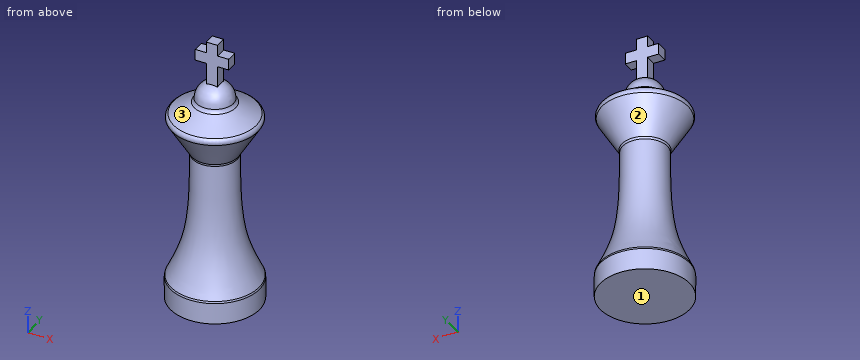
from build123d import *

# Parameters (mm, degrees)
F0_W     = 5
F0_H     = 20
F1_DEPTH = 2.5
F2_W     = 15
F2_H     = 5
F3_DEPTH = 2.5
F6_DEPTH = 2.5
F7_DEPTH = 5
F8_R     = 2


with BuildPart() as f1:
    # F0 (on Front) → F1 (new body)
    with BuildSketch(Plane.XZ):
        with Locations((0, 110)):
            Rectangle(F0_W, F0_H)
    extrude(amount=F1_DEPTH)

    # F2 (on face) → F3 (join)
    with BuildSketch(Plane.XZ.offset(2.5)):
        with Locations((0, 112.5)):
            Rectangle(F2_W, F2_H)
    extrude(amount=-F3_DEPTH)

    # F4 (on Front) → F5 (revolve)
    with BuildSketch(Plane.XZ):
        with BuildLine():
            ThreePointArc((0, 101), (-6.2047476742, 98.408443436), (-8.2411444559, 92))
            Line((-8.2411444559, 92), (-20.3046236384, 85))
            Line((-20.3046236384, 85), (-10, 68))
            add(Edge.make_bspline(
                [(-10, 68), (-10.0457358367, 54.4372630993), (-10.1262334968, 30.5660788152), (-17.0221094404, 16.2026514332), (-20, 10)],
                knots=[0, 0, 0, 0, 0.568163554, 1, 1, 1, 1], degree=3))
            Line((-20, 10), (-20, 0))
            Line((-20, 0), (0, 0))
            Line((0, 0), (0, 101))
        make_face()
    revolve(axis=Axis((0, 0, 50.5), (0, 0, -1)))

    # F0 (on Front) → F6 (join)
    with BuildSketch(Plane.XZ):
        with Locations((0, 110)):
            Rectangle(F0_W, F0_H)
    extrude(amount=-F6_DEPTH)

    # F2 (on face) → F7 (join)
    with BuildSketch(Plane.XZ.offset(2.5)):
        with Locations((0, 112.5)):
            Rectangle(F2_W, F2_H)
    extrude(amount=-F7_DEPTH)

    # F8
    f8_edges = [f1.edges().sort_by_distance(p)[0] for p in [
        (20.304624, 0, 85),
        (20, 0, 10),
        (10, 0, 68),
        (8.241144, 0, 92),
    ]]
    fillet(f8_edges, radius=F8_R)


solid = f1.part
Check sheet for the modelled part. Datum: model origin and axes. Units: mm. Face numbers are marked on the shaded views. Round coordinates to 2 decimals unless told otherwise and drop trailing zeros. Loops run counter-clockwise (first coordinate to the right, second up) from the corner with the lowest first, then second, coordinate; pieces in that order, holes last.
1. Sectioned sample at A-A on z = 81. Record the boundary of the cut face in (x, y), and give its area (3 significant figures).
2. Mould release check, pull along Z, two halves, no side actions. Record for the marked faces 1, 2 and 3: released by +Z, released by -Z, zero draft, split by the parting line, or undercut.
3. Gauge pin test, flat ends, axial feed: pin 1 Ø1.5 at (y, z) = (-0.5, 118) entering from -X; pin 2 Ø2.5 at (y, z) = (-0.5, 111.5) entering from +X; pin 3 Ø2.5 at (x, y) = (4.5, -0.5) entering from +Z. Record the tip position at first contact, or that the pin passes through.
4. Scan lines: probe 1 along Z at (x, y) = (14, 10); probe 2 along Z at (x, y) = (-15, -13); probe 3 along Z at (x, y) = (18.5, 2). Record each from-to range of solid material in increasing order.
Recorded:
1. outline: circle Ø35.76 at (0, 0)
1. area: 1,000 mm2
2. face 1: released by -Z
2. face 2: undercut
2. face 3: released by +Z
3. pin 1: stops at x = -2.5
3. pin 2: stops at x = 7.5
3. pin 3: stops at z = 115
4. probe 1: z = 0 to 15.96, 79.89 to 86.8
4. probe 2: z = 0 to 10.31
4. probe 3: z = 0 to 12.92, 82.2 to 85.98
